```python
from build123d import *

# Parameters (mm, degrees)
EXTRUDE1_DEPTH = 15
SKETCH2_W      = 50
SKETCH2_H      = 130
EXTRUDE2_DEPTH = 10
FILLET1_R      = 10
SKETCH3_W      = 30
SKETCH3_H      = 48.133793791
EXTRUDE3_DEPTH = 8
SKETCH4_W      = 15
SKETCH4_H      = 3.631833837
EXTRUDE4_DEPTH = 48.133793792


with BuildPart() as part:
    # Sketch1 → Extrude1 (new body)
    with BuildSketch(Plane.XY):
        with BuildLine():
            Line((50, 198.565015772), (-20, 198.565015772))
            ThreePointArc((-20, 198.565015772), (-33.5, 212.065015772), (-20, 225.565015772))
            Line((-20, 225.565015772), (50, 225.565015772))
            ThreePointArc((50, 225.565015772), (63.5, 212.065015772), (50, 198.565015772))
        make_face()
    extrude(amount=EXTRUDE1_DEPTH)

    # Sketch2 → Extrude2 (add)
    with BuildSketch(Plane.XY.offset(15)):
        with Locations((15, 160.565015772)):
            Rectangle(SKETCH2_W, SKETCH2_H)
    extrude(amount=EXTRUDE2_DEPTH)

    # Fillet1
    fillet1_edges = [part.edges().sort_by_distance(p)[0] for p in [
        (40, 160.565015772, 25),
        (-10, 160.565015772, 25),
        (15, 225.565015772, 25),
    ]]
    fillet(fillet1_edges, radius=FILLET1_R - 0.0001)  # a hair under: the kernel refuses the full size

    # Sketch3 → Extrude3 (cut)
    with BuildSketch(Plane.XY.offset(25)):
        with Locations((15, 119.631912668)):
            Rectangle(SKETCH3_W, SKETCH3_H)
    extrude(amount=-EXTRUDE3_DEPTH, mode=Mode.SUBTRACT)

    # Sketch4 → Extrude4 (add)
    with BuildSketch(Plane.XZ.offset(-143.698809563)):
        Polygon((30, 17), (30, 25), (15, 25), (0, 25), (0, 17), align=None)
        with Locations((22.5, 26.815916919)):
            Rectangle(SKETCH4_W, SKETCH4_H)
        with Locations((7.5, 26.815916919)):
            Rectangle(SKETCH4_W, SKETCH4_H)
        Polygon((0, 25), (0, 28.631833837), (-15.741772737, 42.308009261), (-15.741772737, 38.676175424), align=None)
        Polygon((45.741772737, 42.308009261), (45.741772737, 38.676175424), (30, 25), (30, 28.631833837), align=None)
    extrude(amount=EXTRUDE4_DEPTH)


solid = part.part
```
Could you check a few things on this model? Use its own coordinates, in mm. A direction names the side the tool comes from. Coordinates: 2 decimals unless noted, no trailing zeros. Order: outer loops, then holes, each group sorted by start corner. A loop starts at its lowest first (then second) coordinate and runs counter-clockwise, first axis right, second up. Notation, with made-up numbers: M 37.25,10.5 L 70.25,10.5 A20 cw 70.25,47.5 Z; hole C -6,54 d5. An arc over 180 degrees is marked long. Use a Markdown table: item, result. Add a question column.
Q1. I want a section at B-B on z = 34. List the corners of the cut face in (x, y) for me, then the cut area to 3 significant figures.
Q2. If I drill on L1, parallel to Z at x = 14.5, y = 156; L2, parallel to Y at x = 35, z = 13.5; L3, parallel to Z at x = 27, y = 211.5, over which ranges is the centre line in solid material (lowest first)?
Q3. Which directions (+Z, -Z, +X, -X, +Y, -Y) give clear straight access to the entire face, cutting with the end or side of a thin tool? Please do faces 1 (the flat face through (15, 183, 25)), 2 (the flat face through (-7.761, 119.969, 35.374)), 3 (the flat face through (37.981, 119.969, 31.934)).
Q4. I'm going to push flat-ended pins straight in: pin 1 (19 mm diameter, centred on x = -23, y = 215, fed in from +Z); pin 2 (24 mm diameter, centred on x = 8, y = 132.5, fed in from +Z); pin 3 (1.1 mm diameter, centred on y = 118.5, z = 40.5, fed in from -X). Where does each tip first touch, or does it pass through?
Q5. We'd pull the mould along Z, two halves only. Please class faces 4 (the flat face through (-7.981, 119.969, 31.934)), 5 (the flat face through (15, 198.565, 7)), 6 (the flat face through (37.761, 119.969, 35.374)): pulls with the +Z half, pulls with the -Z half, needs draft (parallel to the pull), parting line crosses it, or undercut.
Q6. I want a section at A-A on x = 16.5. List the corners of the cut face in (y, z) for me, then the cut area to 3 significant figures.
Q7. I want a section at D-D on x = 44. List the corners of the cut face in (y, z) for me.
Checked values:
| question | item | result |
|---|---|---|
| 1 | outline | M -10.36,95.57 L -6.18,95.57 L -6.18,143.7 L -10.36,143.7 Z; M 36.18,95.57 L 40.36,95.57 L 40.36,143.7 L 36.18,143.7 Z |
| 1 | area | 402 mm² |
| 2 | L1 | 15 to 25 |
| 2 | L2 | 198.57 to 225.57 |
| 2 | L3 | 0 to 25 |
| 3 | face 1 | +Z, +X, -X, +Y |
| 3 | face 2 | +Z, +Y, -Y |
| 3 | face 3 | +X, +Y, -Y |
| 4 | pin 1 | z = 15 |
| 4 | pin 2 | z = 32.11 |
| 4 | pin 3 | x = -15.74 |
| 5 | face 4 | undercut |
| 5 | face 5 | needs draft |
| 5 | face 6 | pulls with the +Z half |
| 6 | outline | M 95.57,15 L 198.57,15 L 198.57,0 L 225.57,0 L 225.57,15 A10 ccw 215.57,25 L 143.7,25 L 143.7,28.63 L 95.57,28.63 Z |
| 6 | area | 1,860 mm² |
| 7 | outline | M 95.57,37.16 L 143.7,37.16 L 143.7,40.79 L 95.57,40.79 Z; M 198.57,0 L 225.57,0 L 225.57,15 L 198.57,15 Z |
